from build123d import *

# Parameters (mm, degrees)
SKETCH1_R           = 24.765
BOSS_EXTRUDE1_DEPTH = 2.286
SKETCH2_R           = 1.7145
SKETCH3_R           = 1.7
CUT_EXTRUDE1_DEPTH  = 36.320159031
CUT_EXTRUDE2_DEPTH  = 36.320159031
CIRPATTERN1_COUNT   = 3
FILLET1_R           = 5
FILLET4_R           = 1
CHAMFER1_SIZE       = 0.5
CHAMFER2_SIZE       = 0.5
CHAMFER3_SIZE       = 0.25


with BuildPart() as part:
    # Sketch1 → Boss-Extrude1 (new, symmetric)
    with BuildSketch(Plane(origin=(0, 0, 0), x_dir=(1, 0, 0), z_dir=(0, 1, 0))):
        with Locations(Location((0, 0, 0), (0, 0, 270))):
            Circle(SKETCH1_R)
    extrude(amount=BOSS_EXTRUDE1_DEPTH, both=True)

    # Sketch2 → Cut-Revolve1 (revolve, cut)
    with BuildSketch(Plane(origin=(0, 0, 0), x_dir=(0, 0, -1), z_dir=(1, 0, 0))):
        with Locations((25.065, 0)):
            Circle(SKETCH2_R)
    revolve(axis=Axis((0, 0, 0), (0, 1, 0)), mode=Mode.SUBTRACT)

    # Sketch3 → Cut-Extrude1 (cut, through all)
    with BuildSketch(Plane(origin=(0, 2.286, 0), x_dir=(1, 0, 0), z_dir=(0, 1, 0))):
        with Locations(Location((0, 0, 0), (0, 0, 270))):
            Circle(SKETCH3_R)
    extrude(amount=-CUT_EXTRUDE1_DEPTH, mode=Mode.SUBTRACT)

    # Sketch4 → Cut-Extrude2 (cut, through all)
    with BuildSketch(Plane(origin=(0, 2.286, 0), x_dir=(1, 0, 0), z_dir=(0, 1, 0))):
        with BuildLine():
            Line((3.742640687, 3.315515147), (17.462152397, 11.236478926))
            ThreePointArc((17.462152397, 11.236478926), (0, 20.765), (-17.462152397, 11.236478926))
            Line((-17.462152397, 11.236478926), (-3.742640687, 3.315515147))
            ThreePointArc((-3.742640687, 3.315515147), (0, 5), (3.742640687, 3.315515147))
        make_face()
    cut_extrude2 = extrude(amount=-CUT_EXTRUDE2_DEPTH, mode=Mode.SUBTRACT)

    # CirPattern1: Cut-Extrude2 ×3 about axis
    cirpattern1_axis = Axis((0, 0, 0), (0, 1, 0))
    for i in range(1, CIRPATTERN1_COUNT):
        add(cut_extrude2.rotate(cirpattern1_axis, i * 360 / CIRPATTERN1_COUNT), mode=Mode.SUBTRACT)

    # Fillet1
    fillet1_edges = [part.edges().sort_by_distance(p)[0] for p in [
        (3.742640687, 0, -3.315515147),
        (-3.742640687, 0, -3.315515147),
        (1, 0, 4.898979486),
        (4.742640687, 0, -1.583464339),
        (-4.742640687, 0, -1.583464339),
        (-1, 0, 4.898979486),
    ]]
    fillet(fillet1_edges, radius=FILLET1_R)

    # Fillet4
    fillet4_edges = [part.edges().sort_by_distance(p)[0] for p in [
        (-17.462152397, 0, -11.236478926),
        (17.462152397, 0, -11.236478926),
        (18.462152397, 0, -9.504428118),
        (1, 0, 20.740907044),
        (-1, 0, 20.740907044),
        (-18.462152397, 0, -9.504428118),
    ]]
    fillet(fillet4_edges, radius=FILLET4_R)

    # Chamfer1
    chamfer1_edges = [part.edges().sort_by_distance(p)[0] for p in [
        (0, -2.286, -1.7),
        (0, 2.286, -1.7),
    ]]
    chamfer(chamfer1_edges, length=CHAMFER1_SIZE)

    # Chamfer2
    chamfer2_edges = [part.edges().sort_by_distance(p)[0] for p in [
        (-17.98301751, 2.286, 10.3825),
        (-17.98301751, -2.286, 10.3825),
        (-11.47866882, 2.286, -7.781913072),
        (-11.47866882, -2.286, -7.781913072),
        (-1, 2.286, 13.831775336),
        (-1, -2.286, 13.831775336),
        (17.006931622, 2.286, -11.354272778),
        (17.006931622, -2.286, -11.354272778),
        (18.336554478, 2.286, -9.051298436),
        (18.336554478, -2.286, -9.051298436),
        (-18.336554478, 2.286, -9.051298436),
        (-18.336554478, -2.286, -9.051298436),
        (-17.006931622, 2.286, -11.354272778),
        (-17.006931622, -2.286, -11.354272778),
        (1.329622856, 2.286, 20.405571214),
        (1.329622856, -2.286, 20.405571214),
        (-1.329622856, 2.286, 20.405571214),
        (-1.329622856, -2.286, 20.405571214),
        (11.47866882, 2.286, -7.781913072),
        (11.47866882, -2.286, -7.781913072),
        (0, 2.286, -5),
        (0, -2.286, -5),
        (4.330127019, 2.286, 2.5),
        (4.330127019, -2.286, 2.5),
        (1, 2.286, 13.831775336),
        (1, -2.286, 13.831775336),
        (-4.330127019, 2.286, 2.5),
        (-4.330127019, -2.286, 2.5),
        (-12.47866882, 2.286, -6.049862264),
        (-12.47866882, -2.286, -6.049862264),
        (4.227779535, 2.286, -4.205135088),
        (4.227779535, -2.286, -4.205135088),
        (-4.227779535, 2.286, -4.205135088),
        (-4.227779535, -2.286, -4.205135088),
        (5.75564358, 2.286, -1.558796935),
        (5.75564358, -2.286, -1.558796935),
        (1.527864045, 2.286, 5.763932023),
        (1.527864045, -2.286, 5.763932023),
        (-1.527864045, 2.286, 5.763932023),
        (-1.527864045, -2.286, 5.763932023),
        (-5.75564358, 2.286, -1.558796935),
        (-5.75564358, -2.286, -1.558796935),
        (0, 2.286, -20.765),
        (0, -2.286, -20.765),
        (12.47866882, 2.286, -6.049862264),
        (12.47866882, -2.286, -6.049862264),
        (17.98301751, 2.286, 10.3825),
        (17.98301751, -2.286, 10.3825),
    ]]
    chamfer(chamfer2_edges, length=CHAMFER2_SIZE)

    # Chamfer3
    chamfer3_edges = [part.edges().sort_by_distance(p)[0] for p in [
        (0, -2.286, -24.765),
        (0, 2.286, -24.765),
    ]]
    chamfer(chamfer3_edges, length=CHAMFER3_SIZE)


solid = part.part
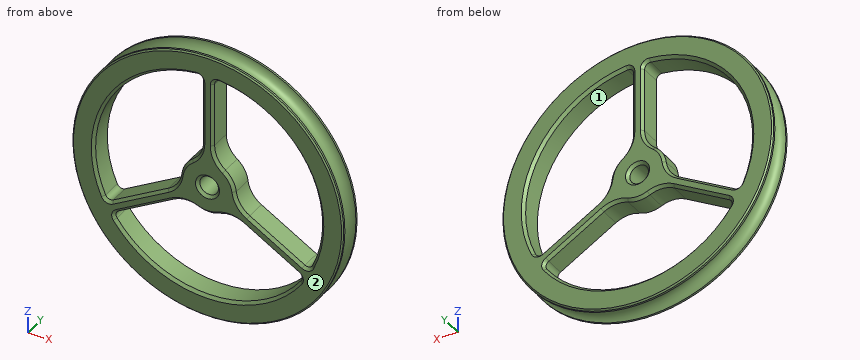
Part model, mm, in its own coordinate system. Face numbers are marked on the shaded views. Coordinates: 2 decimals unless noted, no trailing zeros. Order: outer loops, then holes, each group sorted by start corner. A loop starts at its lowest first (then second) coordinate and runs counter-clockwise, first axis right, second up.
(1) Slice it at B-B, the plane x = 15. State how many separate pieces and enclosed holes the cut face has, and give its area (3 significant figures).
Check sheet entries:
separate pieces: 3
enclosed holes: 0
area: 48.8 mm2
(2) Pin check, flat tips, straight feed: pin 1 Ø2 at (y, z) = (-0.5, 18.5) entering from -X; pin 2 Ø1 at (y, z) = (-1, -3) entering from +X; pin 3 Ø2 at (x, y) = (4.5, 1.5) entering from +Z. Stop position of each tip, or through.
Check sheet entries:
pin 1: stops at x = -15.92
pin 2: stops at x = 24.05
pin 3: stops at z = 24.51
(3) Probe L1, parallel to X at y = 0.4, z = 0 (3 decimals); L2, parallel to X at y = 1.05, z = 13.5; L3, parallel to X at y = 0.4, z = -7. List the from-to ranges inside material, lowest first.
Check sheet entries:
L1: x = -23.398 to -20.765, -5.073 to -1.7, 1.7 to 5.073, 20.765 to 23.398
L2: x = -19.49 to -15.78, -1 to 1, 15.78 to 19.49
L3: x = -22.33 to -19.55, -14.12 to -10.12, 10.12 to 14.12, 19.55 to 22.33
(4) Pull direction Z, two halves, no side cores. Call the marked faces 1 and 2: pulls with the +Z half, pulls with the -Z half, needs draft (parallel to the pull), parting line crosses it, or undercut.
Check sheet entries:
face 1: undercut
face 2: needs draft
(5) Slice it at A-A, the plane y = -0.8. Write the cut outline in (x, z) (3 decimals).
Check sheet entries:
outline: circle Ø47.097 at (0, 0); hole (-18.941, -8.51) arc R1 ccw to (-17.529, -8.966) - (-7.428, -3.134) arc R5 ccw to (-4.964, 0.598) arc R5 cw to (-3, 4) arc R5 ccw to (-1, 8) - (-1, 19.664) arc R1 ccw to (-2.101, 20.658) arc R20.765 ccw to start; hole (-16.84, -12.149) arc R20.765 ccw to (16.84, -12.149) arc R1 ccw to (16.529, -10.698) - (6.428, -4.866) arc R5 ccw to (1.964, -4.598) arc R5 cw to (-1.964, -4.598) arc R5 ccw to (-6.428, -4.866) - (-16.529, -10.698) arc R1 ccw to start; hole circle Ø3.4 at (0, 0); hole (1, 8) arc R5 ccw to (3, 4) arc R5 cw to (4.964, 0.598) arc R5 ccw to (7.428, -3.134) - (17.529, -8.966) arc R1 ccw to (18.941, -8.51) arc R20.765 ccw to (2.101, 20.658) arc R1 ccw to (1, 19.664) - close
